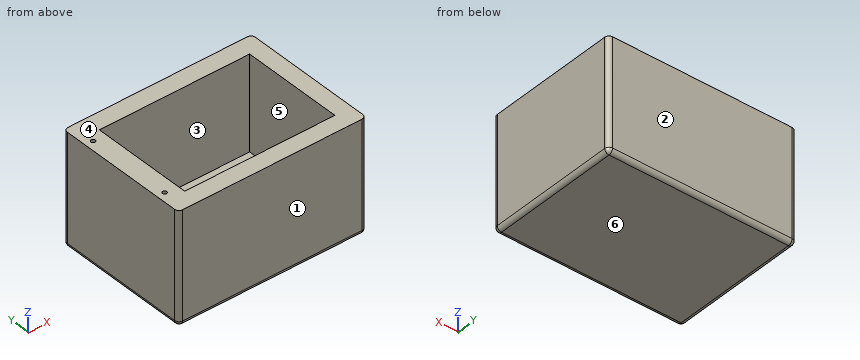
from build123d import *

# Parameters (mm, degrees)
SKETCH_1_W          = 440
SKETCH_1_H          = 320
EXTRUDE_1_DEPTH     = 260
SKETCH_6_W          = 351.529236831
SKETCH_6_H          = 238.132708821
CUT_EXTRUDE_1_DEPTH = 220
FILLET_1_R          = 10
SKETCH_7_R          = 5
CUT_EXTRUDE_2_DEPTH = 10


with BuildPart() as part:
    # 草图1 → 凸台-拉伸1 (new body)
    with BuildSketch(Plane.XY):
        with Locations((220, -160)):
            Rectangle(SKETCH_1_W, SKETCH_1_H)
    extrude(amount=EXTRUDE_1_DEPTH)

    # 草图6 → 切除-拉伸1 (cut)
    with BuildSketch(Plane.XY.offset(260)):
        with Locations((224.235381585, -160.93364559)):
            Rectangle(SKETCH_6_W, SKETCH_6_H)
    extrude(amount=-CUT_EXTRUDE_1_DEPTH, mode=Mode.SUBTRACT)

    # 圆角1
    fillet_1_edges = [part.edges().sort_by_distance(p)[0] for p in [
        (220, 0, 0),
        (440, -160, 0),
        (220, -320, 0),
        (0, -160, 0),
        (0, 0, 130),
        (440, 0, 130),
        (440, -320, 130),
        (0, -320, 130),
    ]]
    fillet(fillet_1_edges, radius=FILLET_1_R)

    # 草图7 → 切除-拉伸2 (cut)
    with BuildSketch(Plane.XY.offset(260)):
        with Locations((18.470763169, -60)):
            Circle(SKETCH_7_R)
        with Locations((18.470763169, -260)):
            Circle(SKETCH_7_R)
    extrude(amount=-CUT_EXTRUDE_2_DEPTH, mode=Mode.SUBTRACT)


solid = part.part
Can you work these out from the model? Positions are in its coordinate system, mm. Face numbers are marked on the shaded views. A direction names the side the tool comes from. Give positions to 0.01 mm unless a question says otherwise; leave off trailing zeros. Order: outer loops, then holes, each group sorted by start corner. A loop starts at its lowest first (then second) coordinate and runs counter-clockwise, first axis right, second up. Notation, with made-up numbers: M -14,29 L 35,29 A15 cw 35,34 Z; hole C -23.75,42 d5. An arc over 180 degrees is marked long. Use one line per item in the form item = value. Start each with the question number.
Item 1: Will these pins go through, and if not, where does the flat tip stop? pin 1 Ø5 at (x, y) = (19, -259.5) entering from +Z; pin 2 Ø2 at (x, y) = (97.5, -190.5) entering from +Z.
Item 2: If we section it at B-B (z = 138.5): Write out the boundary of the cut face in (x, y), then the cut area to 3 significant figures.
Item 3: If we section it at D-D (y = -186): Write out the boundary of the cut face in (x, z).
Item 4: If we section it at A-A (y = -60): Write out the boundary of the cut face in (x, z), then the cut area to 3 significant figures.
Item 5: If I drill on line 1 along X through (y, z) = (-260, 254); line 2 along X through (y, z) = (-228, 123); line 3 along Y through (x, z) = (53.5, 53), over which ranges is the centre line in solid material (lowest first)?
Item 6: We'd pull the mould along Y, two halves only. Please class the marked faces 1, 2, 3 and 4: +Y half, -Y half, draft (parallel to the pull), parting line (faces both ways), or undercut.
Item 7: For the marked faces 5 and 6, which set-ups out of +Z, -Z, +X, -X, +Y, -Y let a thin tool reach every point of the face, with its end or its side?
Item 8: If we section it at C-C (x = 333): Write out the boundary of the cut face in (y, z).
Outcome:
q1.pin_1 = 250
q1.pin_2 = 40
q2.outline = M 0,-310 A10 ccw 10,-320 L 430,-320 A10 ccw 440,-310 L 440,-10 A10 ccw 430,0 L 10,0 A10 ccw 0,-10 Z; hole M 48.47,-280 L 400,-280 L 400,-41.87 L 48.47,-41.87 Z
q2.area = 57,000 mm2
q3.outline = M 0,10 A10 ccw 10,0 L 430,0 A10 ccw 440,10 L 440,260 L 400,260 L 400,40 L 48.47,40 L 48.47,260 L 0,260 Z
q4.outline = M 0,10 A10 ccw 10,0 L 430,0 A10 ccw 440,10 L 440,260 L 400,260 L 400,40 L 48.47,40 L 48.47,260 L 23.47,260 L 23.47,250 L 13.47,250 L 13.47,260 L 0,260 Z
q4.area = 36,900 mm2
q5.line_1 = 0 to 13.47, 23.47 to 48.47, 400 to 440
q5.line_2 = 0 to 48.47, 400 to 440
q5.line_3 = -320 to -280, -41.87 to 0
q6.face_1 = -Y half
q6.face_2 = +Y half
q6.face_3 = undercut
q6.face_4 = draft
q7.face_5 = +Z
q7.face_6 = -Z, +X, -X, +Y, -Y
q8.outline = M -320,10 A10 ccw -310,0 L -10,0 A10 ccw 0,10 L 0,260 L -41.87,260 L -41.87,40 L -280,40 L -280,260 L -320,260 Z
